from build123d import *

# Parameters (mm, degrees)
BOSS_EXTRUDE1_DEPTH = 150
SKETCH2_W           = 75
SKETCH2_H           = 50
BOSS_EXTRUDE2_DEPTH = 50
SKETCH3_R           = 12.5
CUT_EXTRUDE1_DEPTH  = 167


with BuildPart() as part:
    # Sketch1 → Boss-Extrude1 (new body)
    with BuildSketch(Plane.XY):
        Polygon((25, 0), (25, 19.336654422), (50, 19.336654422), (50, 0), (75, 0), (75, -400), (50, -400), (50, -419.336654422), (25, -419.336654422), (25, -400), (0, -400), (0, 0), align=None)
    extrude(amount=BOSS_EXTRUDE1_DEPTH)

    # Sketch2 → Boss-Extrude2 (add)
    with BuildSketch(Plane.XY.offset(150)):
        with Locations((37.5, -205.663345578)):
            Rectangle(SKETCH2_W, SKETCH2_H)
    extrude(amount=BOSS_EXTRUDE2_DEPTH)

    # Sketch3 → Cut-Extrude1 (cut)
    with BuildSketch(Plane.ZY):
        with Locations(Location((175, -205.663345578, 0), (0, 0, 270))):
            Circle(SKETCH3_R)
    extrude(amount=-CUT_EXTRUDE1_DEPTH, mode=Mode.SUBTRACT)


solid = part.part
Can you work these out from the model? Positions are in its coordinate system, mm. A direction names the side the tool comes from. Coordinates: 2 decimals unless noted, no trailing zeros. Loops run counter-clockwise (first coordinate to the right, second up) from the corner with the lowest first, then second, coordinate; pieces in that order, holes last. Notation, with made-up numbers: (21, 46.5) - (25, 46.5) arc R21 ccw to (25, 74.5) - close; hole circle Ø6 at (53, 88.25). An arc over 180 degrees is marked (long way). Put each result on its own line as item: value. Start each with the question number.
Item 1: For pin 1 (22.5 mm diameter, centred on x = 24, y = -298.5, fed in from +Z); pin 2 (10 mm diameter, centred on x = 58, z = 73, fed in from +Y); pin 3 (21.5 mm diameter, centred on y = -412, z = 50.5, fed in from -X); pin 4 (15.5 mm diameter, centred on y = 6.5, z = 52.5, fed in from +X), each with a flat end and sliding along its axis, tell me the tip position at first contact or that it passes through.
Item 2: Suppose I cut it at B-B (x = 57). Please give me the cut outline in (y, z), and give its area (3 significant figures).
Item 3: Suppose I cut it at C-C (z = 23). Please give me the cut outline in (x, y), and give its area (3 significant figures).
Item 4: If we mould it in two halves opening along Y, with no side actions, what happens to faces 5 (the face through (62, 0, 74)), 6 (the face through (38, -419.337, 74)), 7 (the face through (36.98, -196.45, 183.45))? For each: +Y half, -Y half, draft (parallel to the pull), parting line (faces both ways), or undercut.
Item 5: If I drill on line 1 along Z through (x, y) = (12.5, -161); line 2 along Y through (x, z) = (11.5, 30); line 3 along Y through (x, z) = (17.5, 155.5), over which ranges is the centre line in solid material (lowest first)?
Item 6: Suppose I cut it at D-D (x = 38). Please give me the cut outline in (y, z).
Item 7: Which directions (+Z, -Z, +X, -X, +Y, -Y) give clear straight access to the entire face, cutting with the end or side of a thin tool? Please do faces 1 (the face through (37, -230.663, 175)), 2 (the face through (25, -410, 74)), 3 (the face through (25, 10, 74)), 4 (the face through (37, -180.663, 175)).
Item 8: Suppose I cut it at A-A (z = 175). Please give me the cut outline in (x, y).
Here are the results:
1. pin 1: z = 150
1. pin 2: y = 0
1. pin 3: x = 25
1. pin 4: x = 75
2. outline: (-400, 0) - (0, 0) - (0, 150) - (-180.66, 150) - (-180.66, 200) - (-230.66, 200) - (-230.66, 150) - (-400, 150) - close; hole circle Ø25 at (-205.66, 175)
2. area: 62,000 mm²
3. outline: (0, -400) - (25, -400) - (25, -419.34) - (50, -419.34) - (50, -400) - (75, -400) - (75, 0) - (50, 0) - (50, 19.34) - (25, 19.34) - (25, 0) - (0, 0) - close
3. area: 31,000 mm²
4. face 5: +Y half
4. face 6: -Y half
4. face 7: undercut
5. line 1: 0 to 150
5. line 2: -400 to 0
5. line 3: -230.66 to -180.66
6. outline: (-419.34, 0) - (19.34, 0) - (19.34, 150) - (-180.66, 150) - (-180.66, 200) - (-230.66, 200) - (-230.66, 150) - (-419.34, 150) - close; hole circle Ø25 at (-205.66, 175)
7. face 1: +Z, +X, -X, -Y
7. face 2: +Z, -Z, -X, -Y
7. face 3: +Z, -Z, -X, +Y
7. face 4: +Z, +X, -X, +Y
8. outline: (0, -230.66) - (75, -230.66) - (75, -218.16) - (0, -218.16) - close; (0, -193.16) - (75, -193.16) - (75, -180.66) - (0, -180.66) - close
